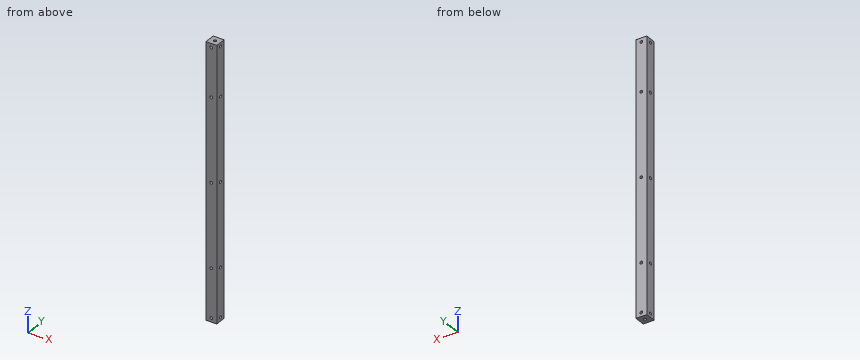
from build123d import *

# Parameters (mm, degrees)
F0_W     = 20
F0_H     = 20
F0_R     = 2.5
F1_DEPTH = 492
F2_R     = 2.5
F3_DEPTH = 20.001
F4_R     = 2.5
F5_DEPTH = 20.001


with BuildPart() as f1:
    # F0 (on Top) → F1 (new body)
    with BuildSketch(Plane.XY):
        Rectangle(F0_W, F0_H)
        Circle(F0_R, mode=Mode.SUBTRACT)
    extrude(amount=F1_DEPTH)

    # F2 (on face) → F3 (cut, through all)
    with BuildSketch(Plane.YZ.offset(10)):
        with Locations((0, 7)):
            Circle(F2_R)
        with Locations((0, 485)):
            Circle(F2_R)
        with Locations((0, 246)):
            Circle(F2_R)
        with Locations((0, 95.127)):
            Circle(F2_R)
        with Locations((0, 396.873)):
            Circle(F2_R)
    extrude(amount=-F3_DEPTH, mode=Mode.SUBTRACT)

    # F4 (on face) → F5 (cut, through all)
    with BuildSketch(Plane.XZ.offset(10)):
        with Locations((0, 246)):
            Circle(F4_R)
        with Locations((0, 485)):
            Circle(F4_R)
        with Locations((0, 7)):
            Circle(F4_R)
        with Locations((0, 95.127)):
            Circle(F4_R)
        with Locations((0, 396.873)):
            Circle(F4_R)
    extrude(amount=-F5_DEPTH, mode=Mode.SUBTRACT)


solid = f1.part
Read the model definition and answer for the solid it produces. Units are mm, in the model's axes. Round coordinates to 2 decimals unless told otherwise and drop trailing zeros. Write each loop counter-clockwise with the first axis right and the second up, starting at its lowest first coordinate (ties: lowest second). Pieces come first, ordered by that corner, then holes. Notation, with made-up numbers: (46.5, 45) - (87.5, 45) arc R21 ccw to (87.5, 70) - close; hole circle Ø4 at (31, 19.5). An arc over 180 degrees is marked (long way). One line per question, with ' | ' between items. Start each with the question number.
1. This flat-tipped pin is pushed along its axis until it touches: pin 1 (4 mm diameter, centred on x = -2, y = 0.5, fed in from -Z). Where does it stop, or does it pass through?
2. Find the intervals of material crossed by probe 1 along Z at (x, y) = (0, -3.25); probe 2 along Z at (x, y) = (-9, -1.75); probe 3 along Y at (x, z) = (0, 58), in increasing order. Write a range as [from, to].
3. Section A-A (z = 79) is taken. Determine the outline of the cut face in (x, y).
Filled in:
1) pin 1: z = 0
2) probe 1: [0, 4.5], [9.5, 92.63], [97.63, 243.5], [248.5, 394.37], [399.37, 482.5], [487.5, 492] | probe 2: [0, 5.21], [8.79, 93.34], [96.91, 244.21], [247.79, 395.09], [398.66, 483.21], [486.79, 492] | probe 3: [-10, -2.5], [2.5, 10]
3) outline: (-10, -10) - (10, -10) - (10, 10) - (-10, 10) - close; hole circle Ø5 at (0, 0)
